from build123d import *

# Parameters (mm, degrees)
EXTRUDE_1_DEPTH      = 30
EXTRUDE_1_DEPTH_BACK = 0.0001
SKETCH_3_R           = 2.5
CUT_EXTRUDE_1_DEPTH  = 20
SKETCH_4_R           = 2.5
EXTRUDE_2_DEPTH      = 8
SKETCH_5_R           = 7.900729049
CUT_EXTRUDE_2_DEPTH  = 2
SKETCH_6_R           = 13.970712395
CUT_EXTRUDE_3_DEPTH  = 10


with BuildPart() as part:
    # 草图2 → 凸台-拉伸1 (new, two sides: drawn at the far end of the back side and taken through both)
    with BuildSketch(Plane(origin=(0, 0, 0), x_dir=(1, 0, 0), z_dir=(0, 1, 0)).offset(-EXTRUDE_1_DEPTH_BACK)):
        Polygon((0, -4.041451884), (3.5, -2.020725942), (3.5, 2.020725942), (0, 4.041451884), (-3.5, 2.020725942), (-3.5, -2.020725942), align=None)
    extrude(amount=EXTRUDE_1_DEPTH + EXTRUDE_1_DEPTH_BACK)

    # 草图3 → 切除-拉伸1 (cut)
    with BuildSketch(Plane.XZ.offset(0.0001)):
        with Locations(Location((0, 0, 0), (0, 0, 270))):
            Circle(SKETCH_3_R)
    extrude(amount=-CUT_EXTRUDE_1_DEPTH, mode=Mode.SUBTRACT)

    # 草图4 → 凸台-拉伸2 (add)
    with BuildSketch(Plane(origin=(0, 30, 0), x_dir=(1, 0, 0), z_dir=(0, 1, 0))):
        with Locations(Location((0, 0, 0), (0, 0, 90))):
            Circle(SKETCH_4_R)
    extrude(amount=EXTRUDE_2_DEPTH)

    # 草图5 → 切除-拉伸2 (cut)
    with BuildSketch(Plane.XZ.offset(0.0001)):
        Circle(SKETCH_5_R)
    extrude(amount=-CUT_EXTRUDE_2_DEPTH, mode=Mode.SUBTRACT)

    # 草图6 → 切除-拉伸3 (cut)
    with BuildSketch(Plane.XZ.offset(-1.9999)):
        with Locations((-3.086044331, 4.465263264)):
            Circle(SKETCH_6_R)
    extrude(amount=-CUT_EXTRUDE_3_DEPTH, mode=Mode.SUBTRACT)


solid = part.part
Geometry: final body of the model. Coordinates: model frame, mm. A direction names the side the tool comes from. Coordinates: 2 decimals unless noted, no trailing zeros. Order: outer loops, then holes, each group sorted by start corner. A loop starts at its lowest first (then second) coordinate and runs counter-clockwise, first axis right, second up.
1) Ray query, probe 1 along X at (y, z) = (16, 0); probe 2 along Y at (x, z) = (-0.25, 1.5); probe 3 along Y at (x, z) = (1.25, -3). Return the intervals inside material, ascending.
Result sheet:
probe 1: x = -3.5 to -2.5, 2.5 to 3.5
probe 2: y = 20 to 38
probe 3: y = 12 to 30
2) Section C-C (y = 23.75). Return loops of the section in (x, z), then the cut area to 3 significant figures.
Result sheet:
outline: (-3.5, -2.02) - (0, -4.04) - (3.5, -2.02) - (3.5, 2.02) - (0, 4.04) - (-3.5, 2.02) - close
area: 42.4 mm2
3) Section A-A (y = 18.5). Return loops of the section in (x, z).
Result sheet:
outline: (-3.5, -2.02) - (0, -4.04) - (3.5, -2.02) - (3.5, 2.02) - (0, 4.04) - (-3.5, 2.02) - close; hole circle Ø5 at (0, 0)
4) Draft query along Z for faces 4 (the cylindrical face through (-2.44, 15.94, 0.54)), 5 (the flat face through (3.5, 21, 0)), 6 (the flat face through (1.8, 20.9, -3)). Return one class per face: released by +Z, released by -Z, zero draft, split by the parting line, or undercut.
Result sheet:
face 4: undercut
face 5: zero draft
face 6: released by -Z
5) First-contact query: P1, Ø1, axis at x = 2.5, z = 2, coming from the +Y side; P2, Ø1, axis at x = 2.5, y = 35, coming from the -Z side; P3, Ø2, axis at x = 1, y = 31.5, coming from the -Z side; P4, Ø4, axis at x = 0.5, z = 0.5, coming from the -Y side. Flat tips, straight axial feed; report the tip coordinate or a pass-through.
Result sheet:
P1: stops at y = 30
P2: stops at z = -1.5
P3: stops at z = -2.5
P4: stops at y = 12
6) Set-up query: faces 1 (the flat face through (-1.726, 20.874, -3.045)), 2 (the flat face through (0, 30, 3)), 3 (the flat face through (0, 20, 0)). Return all of +Z, -Z, +X, -X, +Y, -Y with unobstructed straight access to the full face (end or side cutting, diameter ignored); none if empty.
Result sheet:
face 1: -Z, -X, +Y, -Y
face 2: +Y
face 3: -Y
7) Section B-B (z = 0). Return loops of the section in (x, y), then the cut area to 3 significant figures.
Result sheet:
outline: (-3.5, 12) - (-2.5, 12) - (-2.5, 20) - (2.5, 20) - (2.5, 12) - (3.5, 12) - (3.5, 30) - (2.5, 30) - (2.5, 38) - (-2.5, 38) - (-2.5, 30) - (-3.5, 30) - close
area: 126 mm2
8) Section D-D (x = -0.5). Return loops of the section in (y, z), then the cut area to 3 significant figures.
Result sheet:
outline: (12, -3.75) - (30, -3.75) - (30, -2.45) - (38, -2.45) - (38, 2.45) - (30, 2.45) - (30, 3.75) - (12, 3.75) - (12, 2.45) - (20, 2.45) - (20, -2.45) - (12, -2.45) - close
area: 135 mm2
